Source: CAD feature listing. Evaluate the final solid. Frame: model axes, mm. Face numbers are marked on the shaded views. A direction names the side the tool comes from. Coordinates: 2 decimals unless noted, no trailing zeros. Order: outer loops, then holes, each group sorted by start corner. A loop starts at its lowest first (then second) coordinate and runs counter-clockwise, first axis right, second up. Notation, with made-up numbers: (59.25, 21.5) -> (118.25, 21.5) arc R30 ccw to (118.25, 51.5) -> close; hole circle Ø1 at (22, 51.5). An arc over 180 degrees is marked (long way). Put each result on its own line as item: value.
from build123d import *

# Parameters (mm, degrees)
EXTRUDE_1_DEPTH     = 6
SKETCH_2_R          = 25.25
SKETCH_2_R_2        = 22.75
CUT_EXTRUDE_1_DEPTH = 3
FILLET_1_R          = 1
FILLET_2_R          = 2
SKETCH_3_R          = 1.35
CUT_EXTRUDE_2_DEPTH = 7
CHAMFER_1_SIZE      = 1.5


with BuildPart() as part:
    # Эскиз1 → Бобышка-Вытянуть1 (new body)
    with BuildSketch(Plane(origin=(0, 0, 0), x_dir=(1, 0, 0), z_dir=(0, 1, 0))):
        with BuildLine():
            ThreePointArc((22.75, 0), (21.291887311, -8.013615586), (17.104458483, -15))
            Line((17.104458483, -15), (30, -15))
            ThreePointArc((30, -15), (34.878409373, 0), (30, 15))
            Line((30, 15), (17.104458483, 15))
            ThreePointArc((17.104458483, 15), (21.291887311, 8.013615586), (22.75, 0))
        make_face()
    extrude(amount=EXTRUDE_1_DEPTH)

    # Эскиз2 → Вырез-Вытянуть1 (cut)
    with BuildSketch(Plane(origin=(0, 6, 0), x_dir=(1, 0, 0), z_dir=(0, 1, 0))):
        Circle(SKETCH_2_R)
        Circle(SKETCH_2_R_2, mode=Mode.SUBTRACT)
    extrude(amount=-CUT_EXTRUDE_1_DEPTH, mode=Mode.SUBTRACT)

    # Скругление1
    fillet_1_edges = [part.edges().sort_by_distance(p)[0] for p in [
        (17.104458483, 1.5, -15),
        (17.104458483, 1.5, 15),
        (20.311634597, 4.5, 15),
        (20.311634597, 4.5, -15),
    ]]
    fillet(fillet_1_edges, radius=FILLET_1_R)

    # Скругление2
    fillet_2_edges = [part.edges().sort_by_distance(p)[0] for p in [
        (30, 3, -15),
        (30, 3, 15),
    ]]
    fillet(fillet_2_edges, radius=FILLET_2_R)

    # Эскиз3 → Вырез-Вытянуть2 (cut, through all)
    with BuildSketch(Plane(origin=(0, 6, 0), x_dir=(1, 0, 0), z_dir=(0, 1, 0))):
        with Locations((29.393876913, 6)):
            Circle(SKETCH_3_R)
        with Locations((29.393876913, -6)):
            Circle(SKETCH_3_R)
    extrude(amount=-CUT_EXTRUDE_2_DEPTH, mode=Mode.SUBTRACT)

    # Фаска1
    chamfer_1_edges = [part.edges().sort_by_distance(p)[0] for p in [
        (28.043876913, 0, -6),
        (28.043876913, 0, 6),
    ]]
    chamfer(chamfer_1_edges, length=CHAMFER_1_SIZE)


solid = part.part
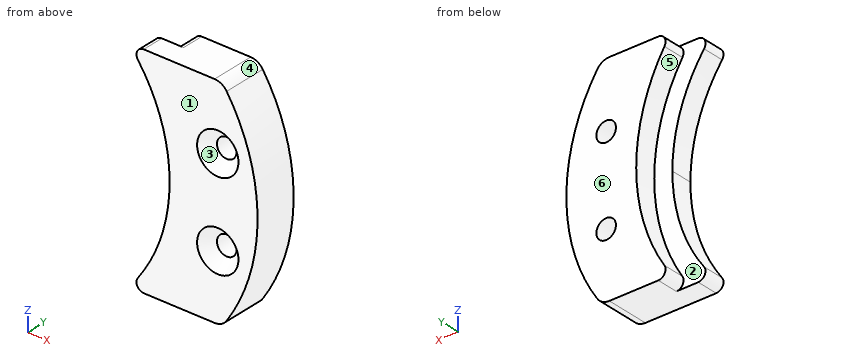
1. Set-up query: the marked faces 1 and 2. Return all of +Z, -Z, +X, -X, +Y, -Y with unobstructed straight access to the full face (end or side cutting, diameter ignored); none if empty.
Numbers:
face 1: +Z, -Z, +X, -X, -Y
face 2: -X, +Y
2. Pull-direction query (X, two-part tool) for the marked faces 3, 4, 5 and 6; classes: pulls with the +X half, pulls with the -X half, needs draft (parallel to the pull), parting line crosses it, or undercut.
Numbers:
face 3: undercut
face 4: pulls with the +X half
face 5: pulls with the -X half
face 6: needs draft
3. First-contact query: pin 1 (2 mm diameter, centred on y = 1, z = -12, fed in from +X); pin 2 (3 mm diameter, centred on y = 5, z = 3, fed in from +X); pin 3 (4.5 mm diameter, centred on x = 29.39, z = -6, fed in from -Y). Flat tips, straight axial feed; report the tip coordinate or a pass-through.
Numbers:
pin 1: stops at x = 32.38
pin 2: stops at x = 34.83
pin 3: stops at y = 0.6
4. Cut plane A-A on y = 2.15. Output: boundary loops of the cut face in (x, z), plus the area to 3 significant figures.
Numbers:
outline: (18.38, -13.41) arc R1 ccw to (19.18, -15) -> (28.96, -15) arc R2 ccw to (30.62, -14.11) arc R25.5 ccw to (30.62, 14.11) arc R2 ccw to (28.96, 15) -> (19.18, 15) arc R1 ccw to (18.38, 13.41) arc R22.75 cw to start; hole circle Ø2.7 at (29.39, -6); hole circle Ø2.7 at (29.39, 6)
area: 357 mm2
5. Cut plane C-C on x = 23.75. Output: boundary loops of the cut face in (y, z), plus the area to 3 significant figures.
Numbers:
outline: (0, -15) -> (6, -15) -> (6, -8.57) -> (3, -8.57) -> (3, 8.57) -> (6, 8.57) -> (6, 15) -> (0, 15) -> close
area: 129 mm2
6. Cut plane D-D on y = 0.6. Output: boundary loops of the cut face in (x, z), plus the area to 3 significant figures.
Numbers:
outline: (18.38, -13.41) arc R1 ccw to (19.18, -15) -> (28.96, -15) arc R2 ccw to (30.62, -14.11) arc R25.5 ccw to (30.62, 14.11) arc R2 ccw to (28.96, 15) -> (19.18, 15) arc R1 ccw to (18.38, 13.41) arc R22.75 cw to start; hole circle Ø4.5 at (29.39, -6); hole circle Ø4.5 at (29.39, 6)
area: 336 mm2
7. Cut plane B-B on z = -6. Output: boundary loops of the cut face in (x, y), plus the area to 3 significant figures.
Numbers:
outline: (21.94, 0) -> (26.54, 0) -> (28.04, 1.5) -> (28.04, 6) -> (24.53, 6) -> (24.53, 3) -> (21.94, 3) -> close; (30.74, 1.5) -> (32.24, 0) -> (34.16, 0) -> (34.16, 6) -> (30.74, 6) -> close
area: 47.1 mm2
8. Ray query, line 1 along Z through (x, y) = (30.25, 1.1); line 2 along Z through (x, y) = (29.5, 3.75); line 3 along Y through (x, z) = (22.75, 4). Return the intervals inside material, ascending.
Numbers:
line 1: z = -14.52 to -7.53, -4.47 to 4.47, 7.53 to 14.52
line 2: z = -14.92 to -7.35, -4.65 to 4.65, 7.35 to 14.92
line 3: y = 0 to 3
